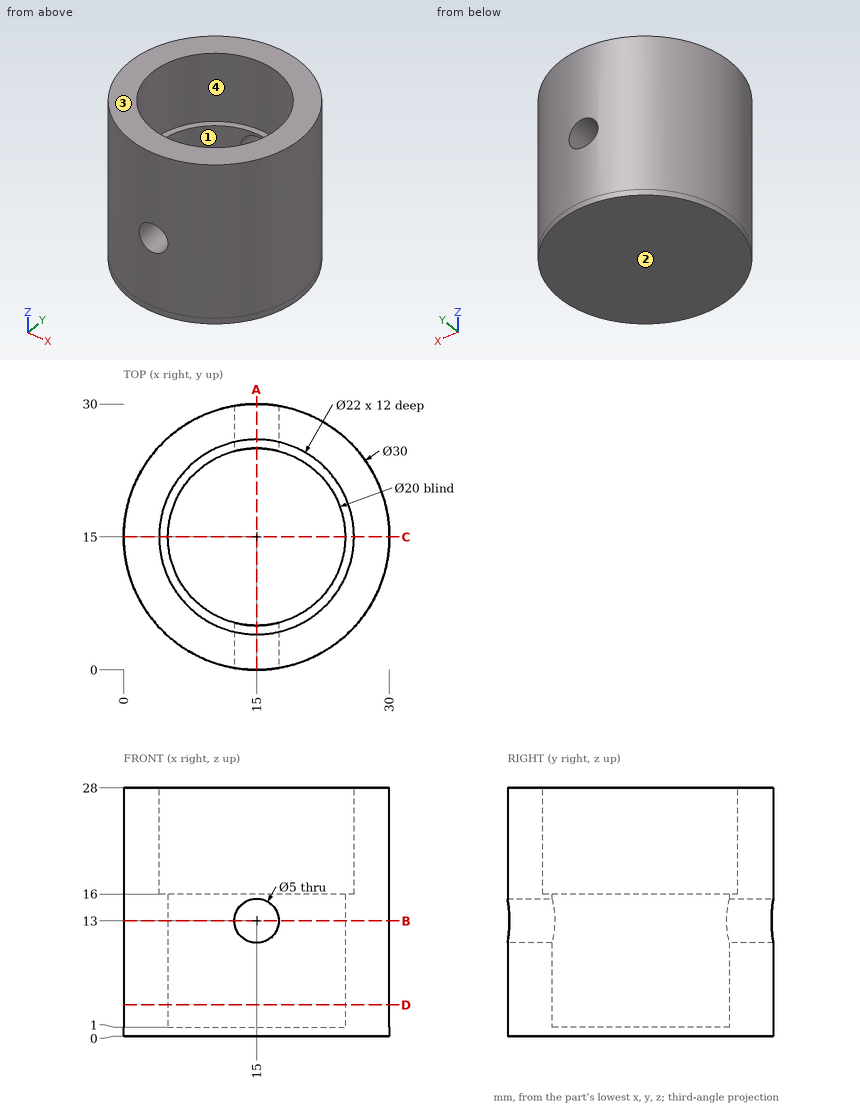
Verification items for this drawing (mm, ordinates from the low corner). A direction names the side the tool comes from. Coordinates: 2 decimals unless noted, no trailing zeros. Order: outer loops, then holes, each group sorted by start corner. A loop starts at its lowest first (then second) coordinate and runs counter-clockwise, first axis right, second up. Notation, with made-up numbers: (-31, 81) -> (9, 81) arc R14 ccw to (9, 86) -> close; hole circle Ø9 at (56, 62.25). An arc over 180 degrees is marked (long way). Put each result on its own line as item: value. Start each with the question number.
1. Go/stop test with flat-tipped pins: pin 1 Ø2 at (x, z) = (16.5, 3.5) entering from -Y; pin 2 Ø17.5 at (x, y) = (12.5, 12) entering from +Z; pin 3 Ø8 at (x, z) = (21, 9.5) entering from -Y; pin 4 Ø5 at (x, z) = (7.5, 24.5) entering from -Y. Record where each tip stops, or that it passes through.
2. Mould release check, pull along Y, two halves, no side actions. Record for the marked faces 3 and 4: released by +Y, released by -Y, zero draft, split by the parting line, or undercut.
3. Access from +Z, -Z, +X, -X, +Y, -Y to the whole of each face (thin tool, end or side, straight path). Record for the marked faces 1 and 2.
4. Cross-section at A-A, the plane x = 15. Record the boundary of the cut face in (y, z).
5. Cross-section at C-C, the plane y = 15. Record the boundary of the cut face in (x, z).
6. Cross-section at B-B, the plane z = 13. Record the boundary of the cut face in (x, y).
7. Cross-section at D-D, the plane z = 3.5. Record the boundary of the cut face in (x, y).
8. Material ranges on L1, parallel to Y at x = 15, z = 5.75; L2, parallel to Y at x = 15, z = 24.5; L3, parallel to Z at x = 20.5, y = 21, recorded low to high. Write a range as [from, to].
Computed:
1. pin 1: y = 0.01
1. pin 2: z = 28
1. pin 3: y = 0.13
1. pin 4: y = 0.86
2. face 3: zero draft
2. face 4: undercut
3. face 1: +Z
3. face 2: -Z, +X, -X, +Y, -Y
4. outline: (0, 0) -> (30, 0) -> (30, 10.5) -> (25, 10.5) -> (25, 1) -> (5, 1) -> (5, 10.5) -> (0, 10.5) -> close; (0, 15.5) -> (5, 15.5) -> (5, 16) -> (4, 16) -> (4, 28) -> (0, 28) -> close; (25, 15.5) -> (30, 15.5) -> (30, 28) -> (26, 28) -> (26, 16) -> (25, 16) -> close
5. outline: (0, 0) -> (30, 0) -> (30, 28) -> (26, 28) -> (26, 16) -> (25, 16) -> (25, 1) -> (5, 1) -> (5, 16) -> (4, 16) -> (4, 28) -> (0, 28) -> close
6. outline: (12.5, 0.21) -> (12.5, 5.32) arc R10 cw to (12.5, 24.68) -> (12.5, 29.79) arc R15 ccw to start; (17.5, 0.21) arc R15 ccw to (17.5, 29.79) -> (17.5, 24.68) arc R10 cw to (17.5, 5.32) -> close
7. outline: circle Ø30 at (15, 15); hole circle Ø20 at (15, 15)
8. L1: [0, 5], [25, 30]
8. L2: [0, 4], [26, 30]
8. L3: [0, 1]
